Here's the drawing with two shaded views (mm, measured from the low corner). I have some questions. A direction names the side the tool comes from. Give positions to 0.01 mm unless a question says otherwise; leave off trailing zeros. Loops run counter-clockwise (first coordinate to the right, second up) from the corner with the lowest first, then second, coordinate; pieces in that order, holes last.
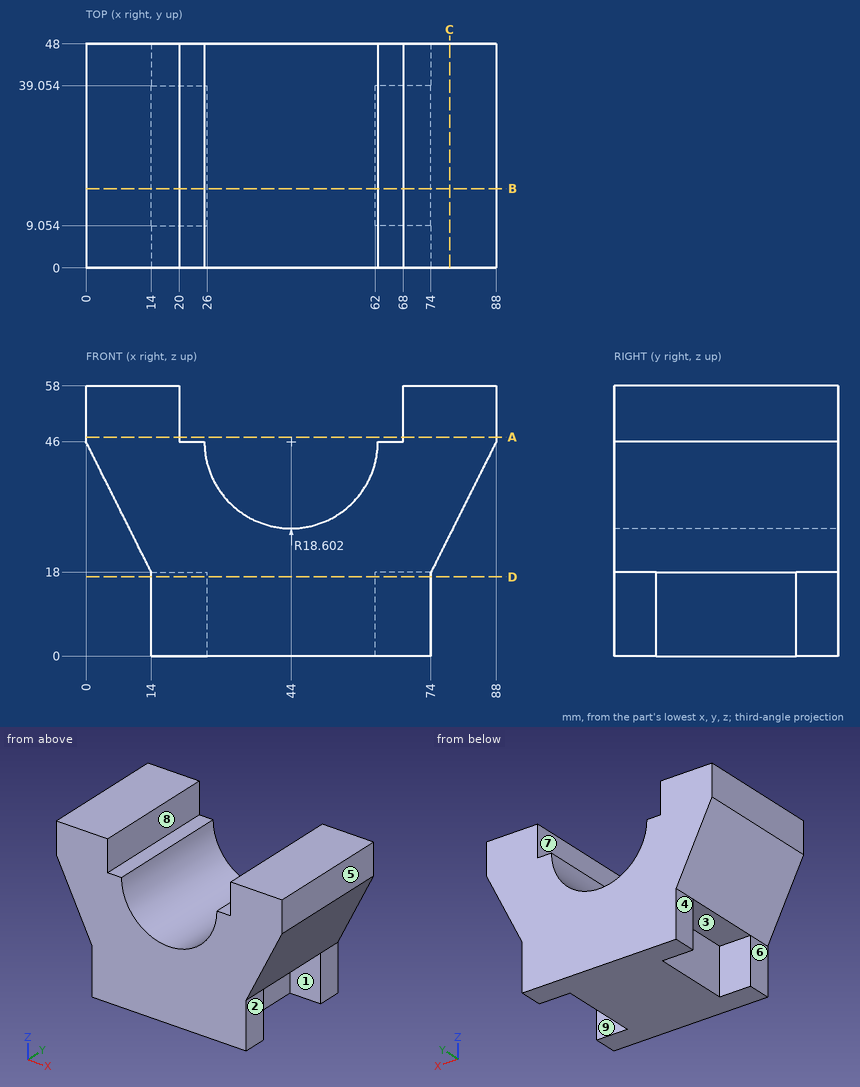
(1) Will these pins go through, and if not, where does the flat tip stop? P1, Ø20, axis at y = 30.5, z = 6, coming from the -X side; P2, Ø10, axis at y = 44, z = 5, coming from the +X side; P3, Ø6, axis at x = 24, y = 27.5, coming from the +Z side.
Returned:
P1: stops at x = 14
P2: stops at x = 74
P3: stops at z = 46
(2) Suppose I cut it at B-B on y = 17. List the corners of the cut face in (x, z) for me.
Returned:
outline: (0, 46) - (14, 18) - (26, 18) - (26, 0) - (62, 0) - (62, 18) - (74, 18) - (88, 46) - (88, 58) - (68, 58) - (68, 46) - (62.6, 46) arc R18.6 cw to (25.4, 46) - (20, 46) - (20, 58) - (0, 58) - close
(3) Which directions (+Z, -Z, +X, -X, +Y, -Y) give clear straight access to the entire face, cutting with the end or side of a thin tool? Please do the marked faces 1, 2, 3, 4 and 5.
Returned:
face 1: -Z, +X
face 2: -Z, +X, +Y, -Y
face 3: -Z, -X
face 4: -Z, -X, +Y, -Y
face 5: +Z, -Z, +X, +Y, -Y
(4) Suppose I cut it at A-A on z = 47. List the corners of the cut face in (x, y) for me, plus the area to 3 significant figures.
Returned:
outline: (0, 0) - (20, 0) - (20, 48) - (0, 48) - close; (68, 0) - (88, 0) - (88, 48) - (68, 48) - close
area: 1,920 mm2
(5) Suppose I cut it at D-D on z = 17. List the corners of the cut face in (x, y) for me (1 decimal), plus the area to 3 significant figures.
Returned:
outline: (14, 0) - (74, 0) - (74, 9.1) - (62, 9.1) - (62, 39.1) - (74, 39.1) - (74, 48) - (14, 48) - (14, 39.1) - (26, 39.1) - (26, 9.1) - (14, 9.1) - close
area: 2,160 mm2
(6) Please list where these lines run through material, in increasing order: probe 1 along X at (y, z) = (28, 52); probe 2 along X at (y, z) = (46.5, 15.5); probe 3 along X at (y, z) = (25, 35).
Returned:
probe 1: x = 0 to 20, 68 to 88
probe 2: x = 14 to 74
probe 3: x = 5.5 to 29, 59 to 82.5
(7) Suppose I cut it at C-C on x = 78. List the corners of the cut face in (y, z) for me.
Returned:
outline: (0, 26) - (48, 26) - (48, 58) - (0, 58) - close
(8) Thinking about a two-plate mould opening in X: for the marked faces 6, 7, 8 and 9, which applies, pulls with the +X half, pulls with the -X half, needs draft (parallel to the pull), parting line crosses it, or undercut?
Returned:
face 6: pulls with the -X half
face 7: undercut
face 8: undercut
face 9: needs draft
